Could you check a few things on this model? Use its own coordinates, in mm. A direction names the side the tool comes from. Give positions to 0.01 mm unless a question says otherwise; leave off trailing zeros. Loops run counter-clockwise (first coordinate to the right, second up) from the corner with the lowest first, then second, coordinate; pieces in that order, holes last. Notation, with made-up numbers: (61, 14) - (102, 14) arc R10 ccw to (102, 31) - close; hole circle Ø8 at (1, 86). An arc over 180 degrees is marked (long way). Use CSV: the item, a comma, the result in double quotes.
from build123d import *

# Parameters (mm, degrees)
F0_W          = 62.5
F0_H          = 36.5
F0_W_2        = 58.5
F0_H_2        = 31.5
F1_DEPTH      = 7
F2_W          = 4
F2_H          = 3
F2_W_2        = 2.1059160829
F2_H_2        = 13
F3_DEPTH      = 1.5
F4_W          = 62.5
F4_H          = 36.5
F5_DEPTH      = 3
F7_DEPTH      = 2.5
F8_R          = 2.5
F9_R          = 1
F11_T1_DEPTH  = 57.5
F11_T3_DEPTH  = 31.5
F11_T6_ANGLE  = 90
F11_T8_ANGLE  = 90
F11_T10_ANGLE = 90
F11_T12_ANGLE = 90
F12_W         = 1.25
F12_H         = 8.5
F13_DEPTH     = 2


# Not quite as in the source:
# - a fillet or chamfer that OpenCascade refuses, or shapes differently, is made with other operations: its cross-section is extruded or revolved along the edge and cut away or added
# - two fillets or chamfers of one size are made in one step


with BuildPart() as f1:
    # F0 (on Top) → F1 (new body)
    with BuildSketch(Plane.XY):
        with Locations((0.5, 0.5)):
            Rectangle(F0_W, F0_H)
        with Locations((1, 0.5)):
            Rectangle(F0_W_2, F0_H_2, mode=Mode.SUBTRACT)
    extrude(amount=F1_DEPTH)

    # F2 (on face) → F3 (join)
    with BuildSketch(Plane.XY.offset(7)):
        Polygon((30.25, 16.25), (-28.25, 16.25), (-28.25, -15.25), (30.25, -15.25), (30.25, -6), (28.1440839171, -6), (5.25, -6), (5.25, 7), (28.1440839171, 7), (30.25, 7), align=None)
        with Locations((-24.25, -7.75)):
            Rectangle(F2_W, F2_H, mode=Mode.SUBTRACT)
        with Locations((-24.25, 8.75)):
            Rectangle(F2_W, F2_H, mode=Mode.SUBTRACT)
        with Locations((29.1970419586, 0.5)):
            Rectangle(F2_W_2, F2_H_2)
    extrude(amount=-F3_DEPTH)

    # F4 (on face) → F5 (join)
    with BuildSketch(Plane(origin=(0, 0, 0), x_dir=(1, 0, 0), z_dir=(0, 0, -1))):
        with Locations((0.5, -0.5)):
            Rectangle(F4_W, F4_H)
        Polygon((-29.5, -17.522141248), (-29.5, 16.5), (30.25, 16.5), (30.25, 15.25), (30.25, -16.25), (30.25, -17.522141248), align=None, mode=Mode.SUBTRACT)
    extrude(amount=F5_DEPTH)

    # F6 (on face) → F7 (cut)
    with BuildSketch(Plane.YZ.offset(-28.25)):
        with BuildLine():
            Line((4, 5.5), (-3, 5.5))
            ThreePointArc((-3, 5.5), (-3.5303300859, 5.2803300859), (-3.75, 4.75))
            Line((-3.75, 4.75), (-3.75, 3.5))
            ThreePointArc((-3.75, 3.5), (-3.1642135624, 2.0857864376), (-1.75, 1.5))
            Line((-1.75, 1.5), (2.75, 1.5))
            ThreePointArc((2.75, 1.5), (4.1642135624, 2.0857864376), (4.75, 3.5))
            Line((4.75, 3.5), (4.75, 4.75))
            ThreePointArc((4.75, 4.75), (4.5303300859, 5.2803300859), (4, 5.5))
        make_face()
    extrude(amount=-F7_DEPTH, mode=Mode.SUBTRACT)

    # F8
    f8_edges = [f1.edges().sort_by_distance(p)[0] for p in [
        (-30.75, 18.75, 2),
        (-30.75, -17.75, 2),
        (31.75, 18.75, 2),
        (31.75, -17.75, 2),
    ]]
    fillet(f8_edges, radius=F8_R)

    # F9
    f9_edges = [f1.edges().sort_by_distance(p)[0] for p in [
        (5.25, 7, 6.25),
        (5.25, -6, 6.25),
        (-22.25, 10.25, 6.25),
        (-22.25, 7.25, 6.25),
        (-26.25, 7.25, 6.25),
        (-26.25, 10.25, 6.25),
        (-26.25, -9.25, 6.25),
        (-26.25, -6.25, 6.25),
        (-22.25, -6.25, 6.25),
        (-22.25, -9.25, 6.25),
    ]]
    fillet(f9_edges, radius=F9_R)

    # F11: fillet of radius 2 on 8 edges, made by hand

    # F11_s2 → F11_t1 (cut)
    with BuildSketch(Plane.YZ.offset(-28.25)):
        with BuildLine():
            ThreePointArc((-15.75, 7), (-17.1642135624, 6.4142135624), (-17.75, 5))
            Line((-17.75, 5), (-17.75, 7))
            Line((-17.75, 7), (-15.75, 7))
        make_face()
        with BuildLine():
            ThreePointArc((16.75, 7), (18.1642135624, 6.4142135624), (18.75, 5))
            Line((18.75, 5), (18.75, 7))
            Line((18.75, 7), (16.75, 7))
        make_face()
    extrude(amount=F11_T1_DEPTH, mode=Mode.SUBTRACT)

    # F11_s4 → F11_t3 (cut)
    with BuildSketch(Plane.XZ.offset(-16.25)):
        with BuildLine():
            ThreePointArc((29.75, 7), (31.1642135624, 6.4142135624), (31.75, 5))
            Line((31.75, 5), (31.75, 7))
            Line((31.75, 7), (29.75, 7))
        make_face()
        with BuildLine():
            ThreePointArc((-28.75, 7), (-30.1642135624, 6.4142135624), (-30.75, 5))
            Line((-30.75, 5), (-30.75, 7))
            Line((-30.75, 7), (-28.75, 7))
        make_face()
    extrude(amount=F11_T3_DEPTH, mode=Mode.SUBTRACT)

    # F11_s5 → F11_t6 (revolve, cut)
    with BuildSketch(Plane.YZ.offset(29.25)):
        with BuildLine():
            ThreePointArc((16.75, 7), (18.1642135624, 6.4142135624), (18.75, 5))
            Line((18.75, 5), (18.75, 7))
            Line((18.75, 7), (16.75, 7))
        make_face()
    revolve(axis=Axis((29.25, 16.25, 7), (0, 0, -1)), revolution_arc=F11_T6_ANGLE, mode=Mode.SUBTRACT)

    # F11_s7 → F11_t8 (revolve, cut)
    with BuildSketch(Plane.YZ.offset(-28.25)):
        with BuildLine():
            ThreePointArc((16.75, 7), (18.1642135624, 6.4142135624), (18.75, 5))
            Line((18.75, 5), (18.75, 7))
            Line((18.75, 7), (16.75, 7))
        make_face()
    revolve(axis=Axis((-28.25, 16.25, 7), (0, 0, 1)), revolution_arc=F11_T8_ANGLE, mode=Mode.SUBTRACT)

    # F11_s9 → F11_t10 (revolve, cut)
    with BuildSketch(Plane.XZ.offset(15.25)):
        with BuildLine():
            ThreePointArc((29.75, 7), (31.1642135624, 6.4142135624), (31.75, 5))
            Line((31.75, 5), (31.75, 7))
            Line((31.75, 7), (29.75, 7))
        make_face()
    revolve(axis=Axis((29.25, -15.25, 7), (0, 0, -1)), revolution_arc=F11_T10_ANGLE, mode=Mode.SUBTRACT)

    # F11_s11 → F11_t12 (revolve, cut)
    with BuildSketch(Plane.XZ.offset(15.25)):
        with BuildLine():
            ThreePointArc((-28.75, 7), (-30.1642135624, 6.4142135624), (-30.75, 5))
            Line((-30.75, 5), (-30.75, 7))
            Line((-30.75, 7), (-28.75, 7))
        make_face()
    revolve(axis=Axis((-28.25, -15.25, 7), (0, 0, 1)), revolution_arc=F11_T12_ANGLE, mode=Mode.SUBTRACT)

    # F12 (on face) → F13 (cut)
    with BuildSketch(Plane(origin=(0, 0, 0), x_dir=(1, 0, 0), z_dir=(0, 0, -1))):
        with Locations((-28.875, -0.5)):
            Rectangle(F12_W, F12_H)
    extrude(amount=-F13_DEPTH, mode=Mode.SUBTRACT)


solid = f1.part
1) We'd pull the mould along X, two halves only. Please class faces 1 (the cylindrical face through (0.1, 18.15, 6.43)), 2 (the cylindrical face through (30.998, -17.037, 1.056)), 3 (the flat face through (5.25, 0, 6)): +X half, -X half, draft (parallel to the pull), parting line (faces both ways), or undercut.
Answer below:
face 1,"draft"
face 2,"+X half"
face 3,"undercut"
2) Which directions (+Z, -Z, +X, -X, +Y, -Y) give clear straight access to the entire face, cutting with the end or side of a thin tool? Please do faces 4 (the flat face through (17, 7, 6)), 5 (the flat face through (0, -16.5, -1)), 6 (the cylindrical face through (-29.76, -3.4, 2.37)).
Answer below:
face 4,"+Z, -Z"
face 5,"-Z"
face 6,"-X"
3) Suppose I cut it at D-D (y = -12.5). Please give me the cut outline in (x, z), plus the area to 3 significant figures.
Answer below:
outline,"(-30.75, -3) - (-29.5, -3) - (-29.5, 0) - (-28.25, 0) - (-28.25, 5.5) - (30.25, 5.5) - (30.25, -3) - (31.75, -3) - (31.75, 5) arc R2 ccw to (29.75, 7) - (-28.75, 7) arc R2 ccw to (-30.75, 5) - close"
area,"122 mm2"
4) Suppose I cut it at A-A (x = 15.5). Please give me the cut outline in (y, z), plus the area to 3 significant figures.
Answer below:
outline,"(-17.75, -3) - (-16.5, -3) - (-16.5, 0) - (-15.25, 0) - (-15.25, 5.5) - (-6, 5.5) - (-6, 7) - (-15.75, 7) arc R2 ccw to (-17.75, 5) - close; (7, 5.5) - (16.25, 5.5) - (16.25, 0) - (17.52, 0) - (17.52, -3) - (18.75, -3) - (18.75, 5) arc R2 ccw to (16.75, 7) - (7, 7) - close"
area,"68.5 mm2"
5) I'm going to push flat-ended pins straight in: P1, Ø0.8, axis at y = 2.5, z = 6, coming from the -X side; P2, Ø0.5, axis at y = 8.5, z = 6, coming from the -X side; P3, Ø1.6, axis at x = -24, z = 6.5, coming from the +Y side. Where does each tip first touch, or does it pass through?
Answer below:
P1,"stops at x = -30.66"
P2,"stops at x = -30.6"
P3,"stops at y = 18.62"
6) Suppose I cut it at B-B (z = -1). Please give me the cut outline in (x, y), plus the area to 3 significant figures.
Answer below:
outline,"(-30.75, -15.25) arc R2.5 ccw to (-28.25, -17.75) - (29.25, -17.75) arc R2.5 ccw to (31.75, -15.25) - (31.75, 16.25) arc R2.5 ccw to (29.25, 18.75) - (-28.25, 18.75) arc R2.5 ccw to (-30.75, 16.25) - close; hole (-29.5, -16.5) - (30.25, -16.5) - (30.25, 17.52) - (-29.5, 17.52) - close"
area,"243 mm2"
7) I need wall thicknesses on line 1 along Y through (x, z) = (-11, 4.75); line 2 along X through (y, z) = (-11.5, 5); line 3 along X through (y, z) = (16.5, -1). Which ranges of each line are inside material? Lowest first, please.
Answer below:
line 1,"y = -17.75 to -15.25, 16.25 to 18.75"
line 2,"x = -30.75 to -28.25, 30.25 to 31.75"
line 3,"x = -30.74 to -29.5, 30.25 to 31.74"
8) Suppose I cut it at C-C (x = -8.5). Please give me the cut outline in (y, z), plus the area to 3 significant figures.
Answer below:
outline,"(-17.75, -3) - (-16.5, -3) - (-16.5, 0) - (-15.25, 0) - (-15.25, 5.5) - (16.25, 5.5) - (16.25, 0) - (17.52, 0) - (17.52, -3) - (18.75, -3) - (18.75, 5) arc R2 ccw to (16.75, 7) - (-15.75, 7) arc R2 ccw to (-17.75, 5) - close"
area,"88.0 mm2"
